Read the model definition and answer for the solid it produces. Units are mm, in the model's axes. A direction names the side the tool comes from. Coordinates: 2 decimals unless noted, no trailing zeros. Write each loop counter-clockwise with the first axis right and the second up, starting at its lowest first coordinate (ties: lowest second). Pieces come first, ordered by that corner, then holes. Notation, with made-up numbers: (-37, 86.5) -> (-19, 86.5) arc R24 cw to (-19, 106.5) -> close; hole circle Ø11 at (85, -36). An arc over 180 degrees is marked (long way). Answer as a JSON object with one key per item and string values. Group by question number.
(1) Find section A-A (z = -3.75). Give the vertices of the cut face in (x, y) (3 decimals).
(2) For a pull along Z with two mould halves and no side action, classify faces 1 (the face through (-2, 0, -15.456)), 2 (the face through (-6, 2, -9.906)), 3 (the face through (-5.524, 1.798, -12.642)), 4 (the face through (-2, 1, 0)) as +Z half, -Z half, draft (parallel to the pull), parting line (faces both ways), or undercut.
(3) Straight lines are drawn through the part: L1, parallel to Z at x = 1.75, y = 3 (3 decimals); L2, parallel to Y at x = -6, z = -7; L3, parallel to Z at x = 3.25, y = 1.25. For each, find the intervals that lie inside material, in ascending order.
(4) Find section B-B (z = -11.25). Count the separate pieces of the cut face and the enclosed holes in it, then the cut area to 3 significant figures.
(5) Flat-ended cylindrical pins translate along their axes: P1, Ø0.5, axis at y = -12.5, z = -7, coming from the -X side; P2, Ø3.5, axis at x = 4.5, y = 2, coming from the +Z side; P3, Ø4, axis at x = -0.5, z = -12.5, coming from the -Y side; P4, Ø1.5, axis at x = 4.85, y = 2.36, coming from the -Z side. Find the tip coordinate at first contact, or state that the pin passes through.
(6) Which of the six approach directions +Z, -Z, +X, -X, +Y, -Y give full straight-line access (tool end or side, diameter ignored) to faces 5 (the face through (-1, 9.271, 1)), 6 (the face through (9.54, -2.9, 2.7)), 7 (the face through (5.23, -5.71, -10.43)), 8 (the face through (6, 3, -9.906)), 9 (the face through (-11.304, -8.008, -6.075))?
from build123d import *

# Parameters (mm, degrees)
BOSS_EXTRUDE1_DEPTH                           = 3.175
BOSS_EXTRUDE2_START                           = -6.858
BOSS_EXTRUDE2_DEPTH                           = 8.5979
BOSS_EXTRUDE3_DEPTH                           = 6.858
CSK_START                                     = -16
CSK_SLOT_FOR_2_FLAT_HEAD_MACHINE_SCREW1_DEPTH = 20
FILLET1_R                                     = 3.175
CHAMFER1_SIZE                                 = 1.5875
F_3_16_0_1875_DIAMETER_HOLE1_D                = 4.7625
F_3_16_0_1875_DIAMETER_HOLE1_DEPTH            = 3.175
F_0_CLEARANCE_HOLE1_D                         = 1.8542
HOLE1_AT_2_COUNT                              = 2
HOLE1_AT_2_PITCH                              = 9.6393
CUT_EXTRUDE2_REACH                            = 30.918
FILLET3_R                                     = 1.5875


with BuildPart() as part:
    # Sketch1 → Boss-Extrude1 (new body)
    with BuildSketch(Plane.XY):
        Polygon((9.9949, 9.271), (9.9949, -15.162995595), (-15.457511269, -16.426312325), (-12.2301, 9.271), align=None)
    extrude(amount=BOSS_EXTRUDE1_DEPTH)



with BuildPart() as body_2:
    # Sketch1<2> → Boss-Extrude2 (new body)
    with BuildSketch(Plane.XY.offset(BOSS_EXTRUDE2_START)):
        Polygon((9.9949, 9.271), (9.9949, -15.162995595), (-15.457511269, -16.426312325), (-12.2301, 9.271), align=None)
    extrude(amount=-BOSS_EXTRUDE2_DEPTH)


with BuildPart() as part_1:
    add(part.part)

    add(body_2.part)  # Boss-Extrude3 merges body 2
    # Sketch3 → Boss-Extrude3 (add)
    with BuildSketch(Plane.XY.offset(-6.858)):
        Polygon((9.9949, -8.812995595), (9.9949, -15.162995595), (-15.457511269, -16.426312325), (-14.501329397, -8.812995595), align=None)
    extrude(amount=BOSS_EXTRUDE3_DEPTH)

    # CSK SLOT for #2 Flat Head Machine Screw1: read off the stored shape, not the designer's step
    # CSK SLOT for _2 Flat Head Machine Sc 2 → CSK SLOT for #2 Flat Head Machine Screw1 (cut)
    with BuildSketch(Plane.XY.offset(CSK_START)):
        with BuildLine():
            Line((-9.342461269, -12.455421191), (-9.342461269, -11.985521191))
            ThreePointArc((-9.342461269, -11.985521191), (-10.695011269, -10.632971191), (-12.047561269, -11.985521191))
            Line((-12.047561269, -11.985521191), (-12.047561269, -12.455421191))
            ThreePointArc((-12.047561269, -12.455421191), (-10.695011269, -13.807971191), (-9.342461269, -12.455421191))
        make_face()
        with BuildLine():
            Line((6.58495, -12.455421191), (6.58495, -11.985521191))
            ThreePointArc((6.58495, -11.985521191), (5.2324, -10.632971191), (3.87985, -11.985521191))
            Line((3.87985, -11.985521191), (3.87985, -12.455421191))
            ThreePointArc((3.87985, -12.455421191), (5.2324, -13.807971191), (6.58495, -12.455421191))
        make_face()
    extrude(amount=CSK_SLOT_FOR_2_FLAT_HEAD_MACHINE_SCREW1_DEPTH, mode=Mode.SUBTRACT)

    # CSK SLOT for _2 Flat Head Machine Sc 3: loft between two sections, ruled curve by curve
    csk_slot_for_2_flat_head_machine_sc_3_from = [
        Edge.make_three_point_arc((-9.342461269, -11.985521191, 2.21806604), (-9.738613992, -11.029123914, 2.21806604), (-10.695011269, -10.632971191, 2.21806604)),
        Edge.make_three_point_arc((-10.695011269, -10.632971191, 2.21806604), (-11.651408546, -11.029123914, 2.21806604), (-12.047561269, -11.985521191, 2.21806604)),
        Edge.make_three_point_arc((-12.047561269, -12.455421191, 2.21806604), (-11.651408546, -13.411818468, 2.21806604), (-10.695011269, -13.807971191, 2.21806604)),
        Edge.make_three_point_arc((-10.695011269, -13.807971191, 2.21806604), (-9.738613992, -13.411818468, 2.21806604), (-9.342461269, -12.455421191, 2.21806604)),
        Edge.make_line((-12.047561269, -11.985521191, 2.21806604), (-12.047561269, -12.455421191, 2.21806604)),
        Edge.make_line((-9.342461269, -11.985521191, 2.21806604), (-9.342461269, -12.455421191, 2.21806604)),
    ]
    csk_slot_for_2_flat_head_machine_sc_3_to = [
        Edge.make_three_point_arc((-8.510611269, -11.985521191, 3.175), (-9.150407216, -10.440917138, 3.175), (-10.695011269, -9.801121191, 3.175)),
        Edge.make_three_point_arc((-10.695011269, -9.801121191, 3.175), (-12.239615322, -10.440917138, 3.175), (-12.879411269, -11.985521191, 3.175)),
        Edge.make_three_point_arc((-12.879411269, -12.455421191, 3.175), (-12.239615322, -14.000025244, 3.175), (-10.695011269, -14.639821191, 3.175)),
        Edge.make_three_point_arc((-10.695011269, -14.639821191, 3.175), (-9.150407216, -14.000025244, 3.175), (-8.510611269, -12.455421191, 3.175)),
        Edge.make_line((-12.879411269, -11.985521191, 3.175), (-12.879411269, -12.455421191, 3.175)),
        Edge.make_line((-8.510611269, -11.985521191, 3.175), (-8.510611269, -12.455421191, 3.175)),
    ]
    csk_slot_for_2_flat_head_machine_sc_3 = Solid(Shell([*[Face.make_surface_from_curves(csk_slot_for_2_flat_head_machine_sc_3_from[k], csk_slot_for_2_flat_head_machine_sc_3_to[k]) for k in range(6)], Face(Wire(csk_slot_for_2_flat_head_machine_sc_3_from)), Face(Wire(csk_slot_for_2_flat_head_machine_sc_3_to))]))
    add(csk_slot_for_2_flat_head_machine_sc_3, mode=Mode.SUBTRACT)

    # CSK SLOT for _2 Flat Head Machine Sc 4: loft between two sections, ruled curve by curve
    csk_slot_for_2_flat_head_machine_sc_4_from = [
        Edge.make_three_point_arc((6.58495, -11.985521191, 2.21806604), (6.188797277, -11.029123914, 2.21806604), (5.2324, -10.632971191, 2.21806604)),
        Edge.make_three_point_arc((5.2324, -10.632971191, 2.21806604), (4.276002723, -11.029123914, 2.21806604), (3.87985, -11.985521191, 2.21806604)),
        Edge.make_three_point_arc((3.87985, -12.455421191, 2.21806604), (4.276002723, -13.411818468, 2.21806604), (5.2324, -13.807971191, 2.21806604)),
        Edge.make_three_point_arc((5.2324, -13.807971191, 2.21806604), (6.188797277, -13.411818468, 2.21806604), (6.58495, -12.455421191, 2.21806604)),
        Edge.make_line((3.87985, -11.985521191, 2.21806604), (3.87985, -12.455421191, 2.21806604)),
        Edge.make_line((6.58495, -11.985521191, 2.21806604), (6.58495, -12.455421191, 2.21806604)),
    ]
    csk_slot_for_2_flat_head_machine_sc_4_to = [
        Edge.make_three_point_arc((7.4168, -11.985521191, 3.175), (6.777004053, -10.440917138, 3.175), (5.2324, -9.801121191, 3.175)),
        Edge.make_three_point_arc((5.2324, -9.801121191, 3.175), (3.687795947, -10.440917138, 3.175), (3.048, -11.985521191, 3.175)),
        Edge.make_three_point_arc((3.048, -12.455421191, 3.175), (3.687795947, -14.000025244, 3.175), (5.2324, -14.639821191, 3.175)),
        Edge.make_three_point_arc((5.2324, -14.639821191, 3.175), (6.777004053, -14.000025244, 3.175), (7.4168, -12.455421191, 3.175)),
        Edge.make_line((3.048, -11.985521191, 3.175), (3.048, -12.455421191, 3.175)),
        Edge.make_line((7.4168, -11.985521191, 3.175), (7.4168, -12.455421191, 3.175)),
    ]
    csk_slot_for_2_flat_head_machine_sc_4 = Solid(Shell([*[Face.make_surface_from_curves(csk_slot_for_2_flat_head_machine_sc_4_from[k], csk_slot_for_2_flat_head_machine_sc_4_to[k]) for k in range(6)], Face(Wire(csk_slot_for_2_flat_head_machine_sc_4_from)), Face(Wire(csk_slot_for_2_flat_head_machine_sc_4_to))]))
    add(csk_slot_for_2_flat_head_machine_sc_4, mode=Mode.SUBTRACT)

    # Fillet1
    fillet1_edges = [part_1.edges().sort_by_distance(p)[0] for p in [
        (-12.2301, 9.271, -11.15695),
        (9.9949, 9.271, -11.15695),
        (9.9949, 9.271, 1.5875),
        (9.9949, -15.162995595, -6.14045),
        (-15.457511269, -16.426312325, -6.14045),
        (-12.2301, 9.271, 1.5875),
    ]]
    fillet(fillet1_edges, radius=FILLET1_R)

    # Chamfer1
    chamfer1_edges = [part_1.edges().sort_by_distance(p)[0] for p in [
        (-2.253214698, -8.812995595, -6.858),
        (-2.253214698, -8.812995595, 0),
    ]]
    chamfer(chamfer1_edges, length=CHAMFER1_SIZE)

    # 3/16 (0.1875) Diameter Hole1
    with Locations(Plane.XY.offset(3.175)):
        with Locations((4.8514, 2.3622), (-4.7879, 2.3622)):
            Hole(F_3_16_0_1875_DIAMETER_HOLE1_D / 2, depth=F_3_16_0_1875_DIAMETER_HOLE1_DEPTH)

    # #0 Clearance Hole1 (through all)
    with Locations(Plane(origin=(0, 0, -15.4559), x_dir=(-1, 0, 0), z_dir=(0, 0, -1))):
        with Locations((-4.8514, 2.3622), (4.7879, 2.3622)):
            Hole(F_0_CLEARANCE_HOLE1_D / 2)

    # Sketch11 → Hole1 (revolve, cut)
    with BuildSketch(Plane(origin=(4.8514, 2.3622, -6.858), x_dir=(0, -1, 0), z_dir=(1, 0, 0))):
        Polygon((0, 0), (0, 3.048), (1.524, 3.048), (1.651, 0), align=None)
    hole1 = revolve(axis=Axis((4.8514, 2.3622, -116.858), (0, 0, 1)), mode=Mode.SUBTRACT)

    # Hole1 at 2: Hole1 ×2
    with Locations(*[(-i * HOLE1_AT_2_PITCH, 0, 0) for i in range(1, HOLE1_AT_2_COUNT)]):
        add(hole1, mode=Mode.SUBTRACT)

    # Sketch13 → Cut-Extrude2 (cut, up to next)
    with BuildSketch(Plane(origin=(0, 0, -15.4559), x_dir=(-1, 0, 0), z_dir=(0, 0, -1)), mode=Mode.PRIVATE) as cut_extrude2_sk1:
        with BuildLine():
            Line((-2.0574, -2.462995595), (6.127656415, -2.462995595))
            ThreePointArc((6.127656415, -2.462995595), (9.302656415, -5.637995595), (6.127656415, -8.812995595))
            Line((6.127656415, -8.812995595), (-2.0574, -8.812995595))
            ThreePointArc((-2.0574, -8.812995595), (-5.2324, -5.637995595), (-2.0574, -2.462995595))
        make_face()
    cut_extrude2_tool1 = extrude(cut_extrude2_sk1.sketch, amount=-CUT_EXTRUDE2_REACH, mode=Mode.PRIVATE) & part_1.part
    add(cut_extrude2_tool1.solids().sort_by_distance((-2.035128, -5.637996, -15.4559))[0], mode=Mode.SUBTRACT)

    # Fillet3
    # the kernel refuses this fillet: 1.5875 mm, written as the material it takes off along each edge
    with BuildSketch(Plane(origin=(-14.985993213, -12.67198858, 3.175), x_dir=(0.9922052502363689, -0.12461437077393937, 0), z_dir=(0.12461437077393936, 0.9922052502363689, 0))) as fillet3_piece_1:
        with BuildLine():
            CenterArc((FILLET3_R, FILLET3_R), FILLET3_R, 180, 90)
            Line((0, FILLET3_R), (0, 0))
            Line((0, 0), (FILLET3_R, 0))
        make_face()
    extrude(amount=19.314188473, mode=Mode.SUBTRACT)
    with BuildSketch(Plane(origin=(-9.4289161, 9.271, 3.175), x_dir=(0, -1, 0), z_dir=(1, 0, 0))) as fillet3_piece_2:
        with BuildLine():
            CenterArc((FILLET3_R, FILLET3_R), FILLET3_R, 180, 90)
            Line((0, FILLET3_R), (0, 0))
            Line((0, 0), (FILLET3_R, 0))
        make_face()
    extrude(amount=16.2488161, mode=Mode.SUBTRACT)
    with BuildSketch(Plane(origin=(6.977295656, -15.312772762, 3.175), x_dir=(-0.04957343510019617, 0.9987704814081995, 0), z_dir=(-0.9987704814081996, -0.049573435100196184, 0))) as fillet3_piece_3:
        with BuildLine():
            CenterArc((FILLET3_R, FILLET3_R), FILLET3_R, 180, 90)
            Line((0, FILLET3_R), (0, 0))
            Line((0, 0), (FILLET3_R, 0))
        make_face()
    extrude(amount=18.678607238, mode=Mode.SUBTRACT)
    with BuildSketch(Plane(origin=(9.9949, 6.096, 3.175), x_dir=(0, 0, -1), z_dir=(0, -1, 0))) as fillet3_piece_4:
        with BuildLine():
            CenterArc((FILLET3_R, -FILLET3_R), FILLET3_R, 90, 90)
            Line((0, -FILLET3_R), (0, 0))
            Line((0, 0), (FILLET3_R, 0))
        make_face()
    extrude(amount=18.237676483, mode=Mode.SUBTRACT)
    with BuildSketch(Plane(origin=(-11.835741543, -13.067639207, 3.175), x_dir=(0.04957343510019569, -0.9987704814081997, 0), z_dir=(0.9987704814081997, 0.04957343510019569, 0))) as fillet3_piece_5:
        with BuildLine():
            CenterArc((3.175 - FILLET3_R, FILLET3_R), FILLET3_R, 270, 90)
            Line((3.175, FILLET3_R), (3.175, 0))
            Line((3.175, 0), (3.175 - FILLET3_R, 0))
        make_face()
    revolve(axis=Axis((-11.835741543, -13.067639207, 3.175), (0, 0, -1)), revolution_arc=100, mode=Mode.SUBTRACT)
    with BuildSketch(Plane(origin=(6.8199, -12.141676483, 3.175), x_dir=(1, 0, 0), z_dir=(0, 1, 0))) as fillet3_piece_6:
        with BuildLine():
            CenterArc((3.175 - FILLET3_R, FILLET3_R), FILLET3_R, 270, 90)
            Line((3.175, FILLET3_R), (3.175, 0))
            Line((3.175, 0), (3.175 - FILLET3_R, 0))
        make_face()
    revolve(axis=Axis((6.8199, -12.141676483, 3.175), (0, 0, -1)), revolution_arc=87.158486733, mode=Mode.SUBTRACT)
    with BuildSketch(Plane(origin=(6.8199, 6.096, 3.175), x_dir=(1, 0, 0), z_dir=(0, -1, 0))) as fillet3_piece_7:
        with BuildLine():
            CenterArc((3.175 - FILLET3_R, -FILLET3_R), FILLET3_R, 0, 90)
            Line((3.175 - FILLET3_R, 0), (3.175, 0))
            Line((3.175, 0), (3.175, -FILLET3_R))
        make_face()
    revolve(axis=Axis((6.8199, 6.096, 3.175), (0, 0, 1)), revolution_arc=90, mode=Mode.SUBTRACT)
    with BuildSketch(Plane(origin=(-9.4289161, 6.096, 3.175), x_dir=(0, 1, 0), z_dir=(1, 0, 0))) as fillet3_piece_8:
        with BuildLine():
            CenterArc((3.175 - FILLET3_R, -FILLET3_R), FILLET3_R, 0, 90)
            Line((3.175, -FILLET3_R), (3.175, 0))
            Line((3.175, 0), (3.175 - FILLET3_R, 0))
        make_face()
    revolve(axis=Axis((-9.4289161, 6.096, 3.175), (0, 0, 1)), revolution_arc=82.841513267, mode=Mode.SUBTRACT)


solid = part_1.part
Results below:
{
 "1": {"outline": "(-14.986, -12.672) arc R3.175 ccw to (-11.678, -16.239) -> (6.977, -15.313) arc R3.175 ccw to (9.995, -12.142) -> (9.995, -8.813) -> (-14.501, -8.813) -> close; hole (-12.048, -12.455) arc R1.353 ccw to (-9.342, -12.455) -> (-9.342, -11.986) arc R1.353 ccw to (-12.048, -11.986) -> close; hole (3.88, -12.455) arc R1.353 ccw to (6.585, -12.455) -> (6.585, -11.986) arc R1.353 ccw to (3.88, -11.986) -> close"},
 "2": {"face 1": "-Z half", "face 2": "+Z half", "face 3": "draft", "face 4": "undercut"},
 "3": {"L1": "z = -15.456 to -6.858, 0 to 3.175", "L2": "y = -15.96 to -8.81, -2.46 to 1.25, 3.47 to 9.27", "L3": "z = -15.46 to -6.86"},
 "4": {"separate pieces": "1", "enclosed holes": "5", "area": "485 mm2"},
 "5": {"P1": "stops at x = -14.99", "P2": "stops at z = -6.86", "P3": "stops at y = -15.78", "P4": "passes through"},
 "6": {"face 5": "+Z, -Z, +X, -X, +Y", "face 6": "+Z, +X, +Y, -Y", "face 7": "-Z", "face 8": "+Z", "face 9": "+X, -X, +Y"}
}
